from build123d import *

# Parameters (mm, degrees)
F0_W          = 25
F0_H          = 25
F1_DEPTH      = 115
F2_W          = 6.9
F2_H          = 9
F3_DEPTH      = 25
F3_DEPTH_BACK = 140
F5_DEPTH      = 26


with BuildPart() as f1:
    # F0 (on Front) → F1 (new body)
    with BuildSketch(Plane.XZ):
        with Locations((4.684485, 2.3731)):
            Rectangle(F0_W, F0_H)
    extrude(amount=F1_DEPTH)

    # F2 (on face) → F3 (join, two sides)
    with BuildSketch(Plane.XZ.offset(115)) as f3_sk:
        with Locations((4.684485, 10.3731)):
            Rectangle(F2_W, F2_H)
    extrude(amount=F3_DEPTH)
    extrude(f3_sk.sketch, amount=-F3_DEPTH_BACK)

    # F4 (on face) → F5 (cut)
    with BuildSketch(Plane.XY.offset(14.8731)):
        with BuildLine():
            ThreePointArc((7.744195, -40), (5.244195, -37.5), (2.744195, -40))
            Line((2.744195, -40), (2.744195, -45))
            ThreePointArc((2.744195, -45), (5.244195, -47.5), (7.744195, -45))
            Line((7.744195, -45), (7.744195, -40))
        make_face()
    extrude(amount=-F5_DEPTH, mode=Mode.SUBTRACT)


solid = f1.part
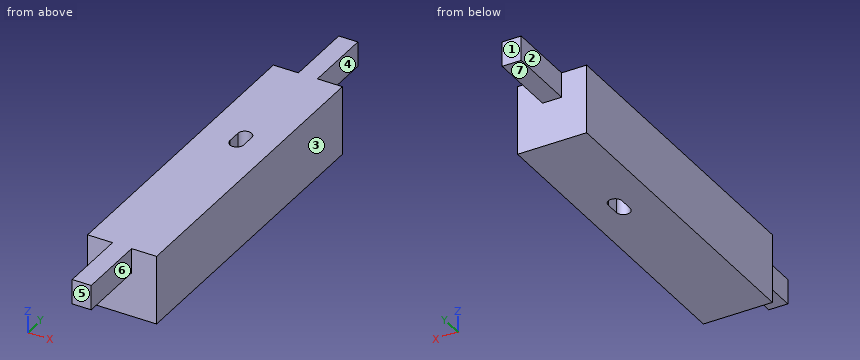
Input: part model. Units: mm. Frame: model coordinates. Face numbers are marked on the shaded views. A direction names the side the tool comes from. Give positions to 0.01 mm unless a question says otherwise; leave off trailing zeros. Order: outer loops, then holes, each group sorted by start corner. A loop starts at its lowest first (then second) coordinate and runs counter-clockwise, first axis right, second up.
Q1. Set-up query: the marked faces 4, 5, 6 and 7. Return all of +Z, -Z, +X, -X, +Y, -Y with unobstructed straight access to the full face (end or side cutting, diameter ignored); none if empty.
Checked values:
face 4: +Z, -Z, +X, +Y
face 5: +Z, -Z, +X, -X, -Y
face 6: +Z, -Z, +X, -Y
face 7: -Z, +X, -X, +Y
Q2. Draft query along X for the marked faces 1, 2 and 3. Return one class per face: +X half, -X half, draft (parallel to the pull), parting line (faces both ways), or undercut.
Checked values:
face 1: draft
face 2: -X half
face 3: +X half
Q3. Section A-A on x = 5. Output: boundary loops of the cut face in (y, z), and give its area (3 significant figures).
Checked values:
outline: (-140, 5.87) - (-115, 5.87) - (-115, -10.13) - (-47.49, -10.13) - (-47.49, 14.87) - (-140, 14.87) - close; (-37.51, -10.13) - (0, -10.13) - (0, 5.87) - (25, 5.87) - (25, 14.87) - (-37.51, 14.87) - close
area: 3,080 mm2
Q4. Ray query, probe 1 along X at (y, z) = (-40, 4.5); probe 2 along Y at (x, z) = (-1.25, -6.5); probe 3 along X at (y, z) = (-46, 11.75). Return the intervals inside material, ascending.
Checked values:
probe 1: x = -7.82 to 2.74, 7.74 to 17.18
probe 2: y = -115 to 0
probe 3: x = -7.82 to 2.95, 7.54 to 17.18
Q5. Section D-D on z = 12.75. Output: boundary loops of the cut face in (x, y), and give its area (3 significant figures).
Checked values:
outline: (-7.82, -115) - (1.23, -115) - (1.23, -140) - (8.13, -140) - (8.13, -115) - (17.18, -115) - (17.18, 0) - (8.13, 0) - (8.13, 25) - (1.23, 25) - (1.23, 0) - (-7.82, 0) - close; hole (2.74, -45) arc R2.5 ccw to (7.74, -45) - (7.74, -40) arc R2.5 ccw to (2.74, -40) - close
area: 3,180 mm2
Q6. Contact query for flat-ended pins moving along their axis: pin 1 Ø2.5 at (y, z) = (8.5, 11.5) entering from +X; pin 2 Ø3.5 at (x, y) = (6, -125.5) entering from -Z; pin 3 Ø5 at (x, z) = (10.5, -3) entering from +Y. Output: stop coordinate, or through.
Checked values:
pin 1: stops at x = 8.13
pin 2: stops at z = 5.87
pin 3: stops at y = 0
Q7. Section C-C on y = 4. Output: boundary loops of the cut face in (x, z).
Checked values:
outline: (1.23, 5.87) - (8.13, 5.87) - (8.13, 14.87) - (1.23, 14.87) - close
Q8. Section B-B on z = -2. Output: boundary loops of the cut face in (x, y).
Checked values:
outline: (-7.82, -115) - (17.18, -115) - (17.18, 0) - (-7.82, 0) - close; hole (2.74, -45) arc R2.5 ccw to (7.74, -45) - (7.74, -40) arc R2.5 ccw to (2.74, -40) - close
